```python
from build123d import *

# Parameters (mm, degrees)
SKETCH1_R           = 10
SKETCH1_R_2         = 4
BOSS_EXTRUDE1_DEPTH = 10
BOSS_EXTRUDE2_DEPTH = 10
SKETCH3_R           = 3
FILLET1_R           = 3


with BuildPart() as part:
    # Sketch1 → Boss-Extrude1 (new body)
    with BuildSketch(Plane(origin=(0, 0, 0), x_dir=(1, 0, 0), z_dir=(0, 1, 0))):
        Circle(SKETCH1_R)
        Circle(SKETCH1_R_2, mode=Mode.SUBTRACT)
    extrude(amount=BOSS_EXTRUDE1_DEPTH)

    # Sketch2 → Boss-Extrude2 (add)
    with BuildSketch(Plane(origin=(0, 10, 0), x_dir=(1, 0, 0), z_dir=(0, 1, 0))):
        with BuildLine():
            Line((-19, -5), (-8.660254038, -5))
            ThreePointArc((-8.660254038, -5), (-10, 0), (-8.660254038, 5))
            Line((-8.660254038, 5), (-19, 5))
            Line((-19, 5), (-19, -5))
        make_face()
    extrude(amount=-BOSS_EXTRUDE2_DEPTH)

    # Sketch3 → Cut-Revolve1 (revolve, cut)
    with BuildSketch(Plane.ZY.offset(19)):
        with Locations((0, 5)):
            Circle(SKETCH3_R)
    revolve(axis=Axis((-19, 10, 5), (0, 0, -1)), mode=Mode.SUBTRACT)

    # Fillet1
    fillet1_edges = [part.edges().sort_by_distance(p)[0] for p in [
        (10, 10, 0),
    ]]
    fillet(fillet1_edges, radius=FILLET1_R)


solid = part.part
```
Work out the finished part from the listing and answer in its coordinate system (mm). Coordinates: 2 decimals unless noted, no trailing zeros. Loops run counter-clockwise (first coordinate to the right, second up) from the corner with the lowest first, then second, coordinate; pieces in that order, holes last. Notation, with made-up numbers: (66, -40) - (79, -40) arc R22 ccw to (79, -18) - close; hole circle Ø5 at (1, -2). An arc over 180 degrees is marked (long way). Use a Markdown table: item, result.
Item 1: Consider probe 1 along Z at (x, y) = (0, 3.25); probe 2 along X at (y, z) = (8.25, 0); probe 3 along X at (y, z) = (4, 1.5). Determine where each line is inside the solid, lowest interval first. Write a range as from..to.
Evaluation:
| item | result |
|---|---|
| probe 1 | z = -10..-4, 4..10 |
| probe 2 | x = -19..-18.03, -11.19..-4, 4..9.73 |
| probe 3 | x = -14.34..-3.71, 3.71..9.89 |
Item 2: Find section B-B, the plane z = -1.75. State how many separate pieces and enclosed holes the cut face has, and give its area (3 significant figures).
Evaluation:
| item | result |
|---|---|
| separate pieces | 3 |
| enclosed holes | 0 |
| area | 176 mm2 |
Item 3: The mould has two halves that part along Z. Classify faces 1 (the flat face through (-19, 7.3, 2.2)), 2 (the cylindrical face through (-0.867, 4.93, 3.905)), 3 (the flat face through (-13, 5, -5)), 4 (the flat face through (-14, 5, 5)): +Z half, -Z half, draft (parallel to the pull), parting line (faces both ways), or undercut.
Evaluation:
| item | result |
|---|---|
| face 1 | draft |
| face 2 | undercut |
| face 3 | -Z half |
| face 4 | +Z half |
Item 4: Find section A-A, the plane x = 0. Determine the outline of the cut face in (y, z).
Evaluation:
| item | result |
|---|---|
| outline | (0, -10) - (7, -10) arc R3 ccw to (10, -7) - (10, -4) - (0, -4) - close; (0, 4) - (10, 4) - (10, 7) arc R3 ccw to (7, 10) - (0, 10) - close |
Item 5: Given pin 1 Ø2 at (x, y) = (-16, 3.5) entering from -Z; pin 2 Ø4 at (x, y) = (-3, 1) entering from -Z; pin 3 Ø3 at (x, y) = (-6.5, 1.5) entering from +Z, each flat-ended and moving along its own axis, determine where each tip first touches the part or whether it passes through.
Evaluation:
| item | result |
|---|---|
| pin 1 | stops at z = -5 |
| pin 2 | stops at z = -9.95 |
| pin 3 | stops at z = 8.66 |
Item 6: Find section C-C, the plane x = -9.75. Determine the outline of the cut face in (y, z), and give its area (3 significant figures).
Evaluation:
| item | result |
|---|---|
| outline | (0, -5) - (10, -5) - (10, 5) - (0, 5) - close |
| area | 100 mm2 |
